Part model, mm, in its own coordinate system. Face numbers are marked on the shaded views. Round coordinates to 2 decimals unless told otherwise and drop trailing zeros. Order: outer loops, then holes, each group sorted by start corner. A loop starts at its lowest first (then second) coordinate and runs counter-clockwise, first axis right, second up. Notation, with made-up numbers: (48, 51) - (57, 51) arc R25 cw to (57, 77) - close; hole circle Ø9 at (78, 1). An arc over 180 degrees is marked (long way). Answer as a JSON object with one key per item and string values.
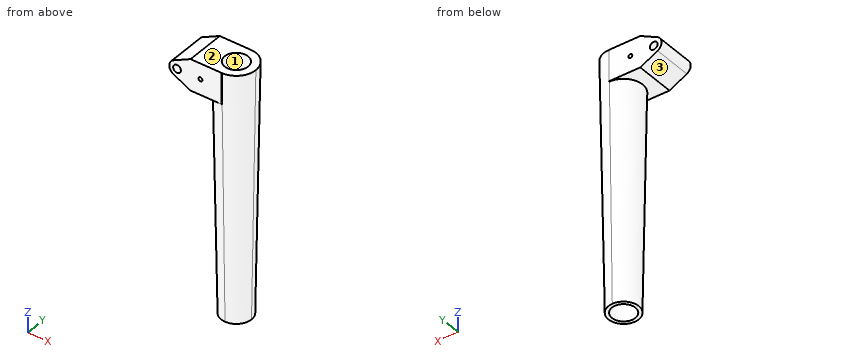
```python
from build123d import *

# Parameters (mm, degrees)
F0_W     = 101.6
F0_H     = 101.6
F0_R     = 12.7
F1_DEPTH = 63.5
F3_DEPTH = 812.8
F3_TAPER = 1
F4_R     = 38.1
F5_DEPTH = 812.8010001
F6_R     = 6.35
F7_DEPTH = 127.0010001


with BuildPart() as f1:
    # F0 (on Front) → F1 (new body, symmetric)
    with BuildSketch(Plane.XZ):
        with Locations((-50.8, 50.8)):
            Rectangle(F0_W, F0_H)
        with BuildLine():
            Line((-158.1918704234, 28.8029547439), (-101.6, 0))
            Line((-101.6, 0), (-101.6, 101.6))
            Line((-101.6, 101.6), (-158.1918704234, 72.7970452561))
            ThreePointArc((-158.1918704234, 72.7970452561), (-170.8918704234, 50.8), (-158.1918704234, 28.8029547439))
        make_face()
        with Locations((-145.4918704234, 50.8)):
            Circle(F0_R, mode=Mode.SUBTRACT)
    extrude(amount=F1_DEPTH, both=True)

    # F2 (on face) → F3 (join)
    with BuildSketch(Plane.XY.offset(101.6)):
        with BuildLine():
            ThreePointArc((0, 63.5), (-63.5, 0), (0, -63.5))
            Line((0, -63.5), (0, 63.5))
        make_face()
        with BuildLine():
            Line((0, 63.5), (0, -63.5))
            ThreePointArc((0, -63.5), (44.9012806053, -44.9012806053), (63.5, 0))
            ThreePointArc((63.5, 0), (44.9012806053, 44.9012806053), (0, 63.5))
        make_face()
    extrude(amount=-F3_DEPTH, taper=F3_TAPER)

    # F4 (on face) → F5 (cut, through all)
    with BuildSketch(Plane.XY.offset(101.6)):
        Circle(F4_R)
    extrude(amount=-F5_DEPTH, mode=Mode.SUBTRACT)

    # F6 (on face) → F7 (cut, through all)
    with BuildSketch(Plane.XZ.offset(63.5)):
        with Locations((-69.2918704234, 50.8)):
            Circle(F6_R)
    extrude(amount=-F7_DEPTH, mode=Mode.SUBTRACT)


solid = f1.part
```
Item 1: Cut at B-B (x = -84.5). Write the cut outline in (y, z).
Taken from the geometry:
{"outline": "(-63.5, 0) - (63.5, 0) - (63.5, 101.6) - (-63.5, 101.6) - close"}
Item 2: Cut at C-C (z = -77). Write the cut outline in (x, y).
Taken from the geometry:
{"outline": "circle Ø120.77 at (0, 0); hole circle Ø76.2 at (0, 0)"}
Item 3: Cut at A-A (y = -21). State how many separate pieces and enclosed holes the cut face has, plus the area to 3 significant figures.
Taken from the geometry:
{"separate pieces": "2", "enclosed holes": "2", "area": "41,600 mm2"}
Item 4: Two-plate mould, pull along X, no slides. Class the marked faces 1, 2 and 3: pulls with the +X half, pulls with the -X half, needs draft (parallel to the pull), parting line crosses it, or undercut.
Taken from the geometry:
{"face 1": "undercut", "face 2": "needs draft", "face 3": "pulls with the -X half"}
Item 5: Probe L1, parallel to X at y = -33, z = 50; L2, parallel to X at y = 4, z = 47; L3, parallel to X at y = -40, z = 56. List the from-to ranges inside material, lowest first. Write a range as from..to.
Taken from the geometry:
{"L1": "-170.88..-158.17, -132.82..-75.59, -62.99..-19.04, 19.04..53.19", "L2": "-170.61..-157.61, -133.37..-74.38, -64.2..-37.89, 37.89..62.42", "L3": "-170.35..-157.08, -133.91..-72.94, -65.65..48.29"}
Item 6: Cut at D-D (z = -582). Write the cut outline in (x, y), plus the area to 3 significant figures.
Taken from the geometry:
{"outline": "circle Ø103.14 at (0, 0); hole circle Ø76.2 at (0, 0)", "area": "3,790 mm2"}
Item 7: Drop flat-ended pins along their axis: P1, Ø5, axis at x = -39.5, z = -79, coming from the +Y side; P2, Ø16.5, axis at x = -69.29, z = 50.8, coming from the +Y side; P3, Ø5, axis at y = -23, z = 16, coming from the +X side; P4, Ø10, axis at x = -125, y = 43, coming from the +Z side. Give the stop position or say it passes through.
Taken from the geometry:
{"P1": "y = 47.68", "P2": "y = 63.5", "P3": "x = 58.52", "P4": "z = 92.24"}
